```python
from build123d import *

# Parameters (mm, degrees)
F1_ANGLE = 180


with BuildPart() as f1:
    # F0 (on Front) → F1 (revolve)
    with BuildSketch(Plane.XZ):
        with BuildLine():
            Line((-39.666668, 64.479168), (-43.458339, 64.479168))
            Line((-43.458339, 64.479168), (-43.458339, 1.979168))
            ThreePointArc((-43.458339, 1.979168), (-42.118593, -3.020832), (-43.458339, -8.020832))
            Line((-43.458339, -8.020832), (-43.458339, -65.520832))
            Line((-43.458339, -65.520832), (-39.666668, -65.520832))
            Line((-39.666668, -65.520832), (-39.666668, -8.020832))
            ThreePointArc((-39.666668, -8.020832), (-38.326922, -3.020832), (-39.666668, 1.979168))
            Line((-39.666668, 1.979168), (-39.666668, 64.479168))
        make_face()
    revolve(axis=Axis((-26.666668, 0, -1.708331), (0, 0, -1)), revolution_arc=F1_ANGLE)


solid = f1.part
```
Could you check a few things on this model? Use its own coordinates, in mm. Coordinates: 2 decimals unless noted, no trailing zeros. Use a Markdown table: item, result. Add a question column.
Q1. We'd pull the mould along X, two halves only. Please class faces 1 (the cylindrical face through (-26.953, 12.997, -36.368)), 2 (the cylindrical face through (-26.953, 12.997, 33.667)), 3 (the flat face through (-41, 0, 0)), 4 (the cylindrical face through (-27.036, 16.788, 32.792)): pulls with the +X half, pulls with the -X half, needs draft (parallel to the pull), parting line crosses it, or undercut.
Q2. I'm going to push flat-ended pins straight in: pin 1 (5 mm diameter, centred on y = 8.5, z = 38, fed in from +X); pin 2 (4 mm diameter, centred on x = -35.5, z = -47.5, fed in from -Y); pin 3 (6 mm diameter, centred on x = -21.5, y = 4, fed in from -Z); pin 4 (8 mm diameter, centred on x = -21.5, z = -47, fed in from +Y). Where does each tip first touch, or does it pass through?
Q3. If I drill on L1, parallel to X at y = 4, z = 2; L2, parallel to X at y = 1.5, z = 52.5; L3, parallel to Y at x = -32, z = -11.5, over which ranges is the centre line in solid material (lowest first)?
Checked values:
| question | item | result |
|---|---|---|
| 1 | face 1 | undercut |
| 1 | face 2 | undercut |
| 1 | face 3 | needs draft |
| 1 | face 4 | parting line crosses it |
| 2 | pin 1 | x = -10.98 |
| 2 | pin 2 | y = 7.19 |
| 2 | pin 3 | through |
| 2 | pin 4 | y = 16.75 |
| 3 | L1 | -42.97 to -39.04, -14.3 to -10.36 |
| 3 | L2 | -43.39 to -39.58, -13.75 to -9.94 |
| 3 | L3 | 11.86 to 15.92 |
